```python
from build123d import *

# Parameters (mm, degrees)
BOSS_EXTRUDE3_DEPTH     = 20
CUT_EXTRUDE1_DEPTH      = 88
CUT_EXTRUDE1_DEPTH_BACK = 161
SKETCH3_R               = 1.7


with BuildPart() as part:
    # Sketch1 → Boss-Extrude3 (new body)
    with BuildSketch(Plane.XY):
        Polygon((0, 0), (65, 0), (65, 20), (9.1, 20), (9.1, 120), (1.6, 120), (1.6, 20), (-1.6, 20), (-1.6, 120), (-9.1, 120), (-9.1, 20), (-65, 20), (-65, 0), align=None)
    extrude(amount=BOSS_EXTRUDE3_DEPTH)

    # Sketch3 → Cut-Extrude1 (cut, two sides: drawn at the far end of the back side and taken through both)
    with BuildSketch(Plane(origin=(9.1, 0, 0), x_dir=(0, 0, -1), z_dir=(1, 0, 0)).offset(-CUT_EXTRUDE1_DEPTH_BACK)):
        with Locations(Location((-10, 95, 0), (0, 0, 180))):
            Circle(SKETCH3_R)
        with Locations(Location((-10, 45, 0), (0, 0, 180))):
            Circle(SKETCH3_R)
    extrude(amount=CUT_EXTRUDE1_DEPTH + CUT_EXTRUDE1_DEPTH_BACK, mode=Mode.SUBTRACT)


solid = part.part
```
Could you check a few things on this model? Use its own coordinates, in mm. A direction names the side the tool comes from. Round coordinates to 2 decimals unless told otherwise and drop trailing zeros. Loops run counter-clockwise (first coordinate to the right, second up) from the corner with the lowest first, then second, coordinate; pieces in that order, holes last. Notation, with made-up numbers: M 73.25,-39 L 78.25,-39 A15 cw 78.25,-34 Z; hole C 68.5,52.25 d10. An arc over 180 degrees is marked long. Put each result on its own line as item: value.
Q1. I need wall thicknesses on probe 1 along Y at (x, z) = (-6.75, 10); probe 2 along X at (y, z) = (41, 18.5); probe 3 along Z at (x, y) = (6, 95). Which ranges of each line are inside material? Lowest first, please.
Check result:
probe 1: 0 to 43.3, 46.7 to 93.3, 96.7 to 120
probe 2: -9.1 to -1.6, 1.6 to 9.1
probe 3: 0 to 8.3, 11.7 to 20
Q2. Imagine slicing it at C-C (y = 45). Write out the boundary of the cut face in (x, z), then the cut area to 3 significant figures.
Check result:
outline: M -9.1,0 L -1.6,0 L -1.6,8.3 L -9.1,8.3 Z; M -9.1,11.7 L -1.6,11.7 L -1.6,20 L -9.1,20 Z; M 1.6,0 L 9.1,0 L 9.1,8.3 L 1.6,8.3 Z; M 1.6,11.7 L 9.1,11.7 L 9.1,20 L 1.6,20 Z
area: 249 mm2
Q3. For pin 1 (1.5 mm diameter, centred on y = 63.5, z = 17, fed in from -X); pin 2 (2 mm diameter, centred on y = 45, z = 10, fed in from +X); pin 3 (4 mm diameter, centred on y = 95, z = 10, fed in from +X); pin 4 (10 mm diameter, centred on x = 29.5, z = 7.5, fed in from +Y), each with a flat end and sliding along its axis, tell me the tip position at first contact or that it passes through.
Check result:
pin 1: x = -9.1
pin 2: through
pin 3: x = 9.1
pin 4: y = 20
Q4. Imagine slicing it at A-A (y = 75.5). Write out the boundary of the cut face in (x, z), then the cut area to 3 significant figures.
Check result:
outline: M -9.1,0 L -1.6,0 L -1.6,20 L -9.1,20 Z; M 1.6,0 L 9.1,0 L 9.1,20 L 1.6,20 Z
area: 300 mm2
Q5. On a 3-axis mill with a long thin cutter (end or side, diameter ignored), from which of +Z, -Z, +X, -X, +Y, -Y can I reach the whole of each face in a straight line? I mean faces 4 (the face through (-5.4, 96.66, 9.63)), 5 (the face through (-1, 0, 10)), 6 (the face through (-9.1, 71, 10)), 7 (the face through (9.1, 69, 10)), 8 (the face through (0, 20, 10)). Say none if no direction works.
Check result:
face 4: +X, -X
face 5: +Z, -Z, +X, -X, -Y
face 6: +Z, -Z, -X, +Y
face 7: +Z, -Z, +X, +Y
face 8: +Z, -Z, +Y
Q6. Imagine slicing it at D-D (z = 17.5). Write out the boundary of the cut face in (x, y).
Check result:
outline: M -65,0 L 65,0 L 65,20 L 9.1,20 L 9.1,120 L 1.6,120 L 1.6,20 L -1.6,20 L -1.6,120 L -9.1,120 L -9.1,20 L -65,20 Z
Q7. Imagine slicing it at B-B (z = 10). Write out the boundary of the cut face in (x, y), then the cut area to 3 significant figures.
Check result:
outline: M -65,0 L 65,0 L 65,20 L 9.1,20 L 9.1,43.3 L 1.6,43.3 L 1.6,20 L -1.6,20 L -1.6,43.3 L -9.1,43.3 L -9.1,20 L -65,20 Z; M -9.1,46.7 L -1.6,46.7 L -1.6,93.3 L -9.1,93.3 Z; M -9.1,96.7 L -1.6,96.7 L -1.6,120 L -9.1,120 Z; M 1.6,46.7 L 9.1,46.7 L 9.1,93.3 L 1.6,93.3 Z; M 1.6,96.7 L 9.1,96.7 L 9.1,120 L 1.6,120 Z
area: 4,000 mm2
Q8. Thinking about a two-plate mould opening in Y: for faces 1 (the face through (-1.6, 69, 10)), 2 (the face through (5, 120, 10)), 3 (the face through (5.3, 96.66, 9.63)), which applies, released by +Y, released by -Y, zero draft, split by the parting line, or undercut?
Check result:
face 1: zero draft
face 2: released by +Y
face 3: undercut
